Model file for the job. Use its own axes, mm. A direction names the side the tool comes from. Round coordinates to 2 decimals unless told otherwise and drop trailing zeros. Write each loop counter-clockwise with the first axis right and the second up, starting at its lowest first coordinate (ties: lowest second). Pieces come first, ordered by that corner, then holes. Notation, with made-up numbers: (-11, -28) - (17, -28) arc R20 ccw to (17, 1) - close; hole circle Ø4 at (58, 87). An arc over 180 degrees is marked (long way). One line per item, written item: value.
Autodesk Inventor part; units mm, degrees
ref_plane "Arbeitsebene1" through (17, 0, 0) normal (1, 0, 0) x (0, 0, -1)
ref_plane "YZ Plane" through (0, 0, 0) normal (1, 0, 0) x (0, 1, 0)
ref_plane "XZ Plane" through (0, 0, 0) normal (0, 1, 0) x (-1, 0, 0)
sketch "Skizze" plane through (0, 0, 0) normal (0, 0, 1) x (1, 0, 0)
  line L0 (0, 0) -> (20, 0)
  line L1 (0, 0) -> (0, 16) construction
  line L2 (0, 16) -> (20, 16)
  line L3 (20, 16) -> (20, 20)
  line L4 (20, 20) -> (0, 20)
  line L5 (0, 20) -> (0, 16)
  dimension "d0" = 32
  dimension "d1" = 40
  dimension "d2" = 20
revolve "Körper" add sketch "Skizze" angle 360 about axis through (0, 0, 0) along (1, 0, 0)
chamfer "Fase1" distance 0.8001 distance2 0.8001 1 edges at (0, -20, 0) measured on face at (0, 18.318, -2.8718)
chamfer "Fase2" distance 0.8001 distance2 0.8001 1 edges at (0, -16, 0) measured on face at (0, 17.7923, -2.808)
chamfer "Fase3" distance 0.8001 distance2 0.8001 1 edges at (20, -16, 0) measured on face at (20, 18.4729, -1.5954)
chamfer "Fase4" distance 0.8001 distance2 0.8001 1 edges at (20, -20, 0) measured on face at (20, 18.7396, -1.5954)
ref_plane "Arbeitsebene1" through (17, 0, 0) normal (1, 0, 0) x (0, 0, -1)
sketch "Skizze2" plane through (17, 0, 0) normal (1, 0, 0) x (0, 0, -1)
  circle A0 centre (0, 0) radius 20
  circle A1 centre (0, 0) radius 18.5
  dimension "d22" = 1.5
  dimension "d23" = 40
extrude "Extrusion1" cut sketch "Skizze2" against normal blind 5
sketch "Skizze3" plane through (0, 0, 0) normal (0, 0, 1) x (1, 0, 0)
  line L0 (12, 20) -> (12, -20)
  line L1 (-4, 0) -> (24, 0)
  point P0 (0, 0)
  point P1 (14.5, 0)
  dimension "d26" = 2.5
hole "Bohrung1" at (14.5, 0, 0) direction (0, 0, -1) diameter 4 depth 35 tip angle 118
equation "\"d0\" = WD"
equation "\"d1\" = BD"
equation "\"d2\" = KB"
equation "\"WD\" = 32"
equation "\"BD\" = 40"
equation "\"KB\" = 20"
equation "\"PHH1\" = 0.8"
equation "\"KID1\" = 33.6"
equation "\"KAD1\" = 38.4"
equation "\"PHH2\" = PHH1"
equation "\"PHH3\" = PHH1"
equation "\"PHH4\" = PHH1"
equation "\"KID2\" = KID1"
equation "\"KAD2\" = KAD1"
equation "\"WR\" = 0.5 * WD"
equation "\"BBA\" = 0"
properties part number "ISO 4379 - 32 x 40 x 20" material "Kupfer, Legierung"
1. Band-saw the part on C-C on x = 6.75. Write the cut outline in (y, z).
Report:
outline: circle Ø40 at (0, 0); hole circle Ø32 at (0, 0)
2. Band-saw the part on A-A on y = 0. Write the cut outline in (x, z).
Report:
outline: (0, -19.2) - (0.8, -20) - (12, -20) - (12, -18.5) - (12.5, -18.5) - (12.5, -16) - (0.8, -16) - (0, -16.8) - close; (0, 16.8) - (0.8, 16) - (19.2, 16) - (20, 16.8) - (20, 19.2) - (19.2, 20) - (17, 20) - (17, 18.5) - (12, 18.5) - (12, 20) - (0.8, 20) - (0, 19.2) - close; (16.5, -18.5) - (17, -18.5) - (17, -20) - (19.2, -20) - (20, -19.2) - (20, -16.8) - (19.2, -16) - (16.5, -16) - close
3. Band-saw the part on D-D on x = 14. Write the cut outline in (y, z).
Report:
outline: (-1.94, -18.4) - (-1.94, -15.88) arc R16 cw (long way) to (1.94, -15.88) - (1.94, -18.4) arc R18.5 ccw (long way) to start
4. Wall check: probe 1 along X at (y, z) = (0, -17.8); probe 2 along Z at (x, y) = (10, 0); probe 3 along Z at (x, y) = (10, -9.5). Give the ranges that are in metal, low to high. Write a range as [from, to].
Report:
probe 1: [0, 12.5], [16.5, 20]
probe 2: [-20, -16], [16, 20]
probe 3: [-17.6, -12.87], [12.87, 17.6]
5. Mould opens along Y. For faces 3 (the face through (12.517, 0.26, -17.205)), 4 (the face through (10.13, -3.47, -15.62)), 5 (the face through (12, -18, -6)), 6 (the face through (18.085, -4.336, 19.524)) say: released by +Y, released by -Y, zero draft, split by the parting line, or undercut.
Report:
face 3: undercut
face 4: undercut
face 5: zero draft
face 6: split by the parting line
6. Drop flat-ended pins along their axis: pin 1 (6 mm diameter, centred on x = 15.5, y = 12, fed in from +Z); pin 2 (12 mm diameter, centred on y = -2, z = -6.5, fed in from +X); pin 3 (6 mm diameter, centred on x = 10.5, y = 13, fed in from +Z); pin 4 (5 mm diameter, centred on x = 7, y = 7.5, fed in from -Z). Give the stop position or say it passes through.
Report:
pin 1: z = 17.65
pin 2: through
pin 3: z = 17.32
pin 4: z = -19.36
7. Tool access for faces 1 (the face through (17, -18, -6)), 2 (the face through (0, 0, -17)): list every direction of +Z, -Z, +X, -X, +Y, -Y with a clear straight run to the whole face (end or side of a thin tool).
Report:
face 1: none
face 2: +Z, -Z, -X, +Y, -Y
8. Band-saw the part on B-B on z = 0. Write the cut outline in (x, y).
Report:
outline: (0, -19.2) - (0.8, -20) - (12, -20) - (12, -18.5) - (17, -18.5) - (17, -20) - (19.2, -20) - (20, -19.2) - (20, -16.8) - (19.2, -16) - (0.8, -16) - (0, -16.8) - close; (0, 16.8) - (0.8, 16) - (19.2, 16) - (20, 16.8) - (20, 19.2) - (19.2, 20) - (17, 20) - (17, 18.5) - (12, 18.5) - (12, 20) - (0.8, 20) - (0, 19.2) - close
